from build123d import *

# Parameters (mm, degrees)
BOSS_EXTRUDE1_DEPTH = 5
FILLET1_R           = 40
FILLET2_R           = 1
SKETCH2_R           = 3
CUT_EXTRUDE1_DEPTH  = 1192.271634267


with BuildPart() as part:
    # Sketch1 → Boss-Extrude1 (new body)
    with BuildSketch(Plane.XY):
        Polygon((0, 0), (230, 0), (600.444279957, 1040), align=None)
    extrude(amount=BOSS_EXTRUDE1_DEPTH)

    # Fillet1
    fillet1_edges = [part.edges().sort_by_distance(p)[0] for p in [
        (230, 0, 2.5),
    ]]
    fillet(fillet1_edges, radius=FILLET1_R)

    # Fillet2
    fillet2_edges = [part.edges().sort_by_distance(p)[0] for p in [
        (600.444279957, 1040, 2.5),
    ]]
    fillet(fillet2_edges, radius=FILLET2_R)

    # Sketch2 → Cut-Extrude1 (cut, through all)
    with BuildSketch(Plane.XY.offset(5)):
        with Locations((249.147691634, 97.758565682)):
            Circle(SKETCH2_R)
        with Locations((273.494533389, 161.250543889)):
            Circle(SKETCH2_R)
        with Locations((515.885480129, 842.044902128)):
            Circle(SKETCH2_R)
        with Locations((540.232321884, 905.536880334)):
            Circle(SKETCH2_R)
    extrude(amount=-CUT_EXTRUDE1_DEPTH, mode=Mode.SUBTRACT)


solid = part.part
Can you work these out from the model? Positions are in its coordinate system, mm. Give positions to 0.01 mm unless a question says otherwise; leave off trailing zeros. Loops run counter-clockwise (first coordinate to the right, second up) from the corner with the lowest first, then second, coordinate; pieces in that order, holes last. Notation, with made-up numbers: (-16, 1) -> (-8, 1) arc R13 ccw to (-8, 21) -> close; hole circle Ø11 at (-8, -19.5). An arc over 180 degrees is marked (long way). Return JSON: item names as keys, results as strings.
Q1. I want a section at C-C, the plane x = 415.5. List the corners of the cut face in (y, z) for me, then the cut area to 3 significant figures.
Checks:
{"outline": "(520.78, 0) -> (719.67, 0) -> (719.67, 5) -> (520.78, 5) -> close", "area": "994 mm2"}
Q2. For pin 1 Ø3.5 at (x, y) = (515.89, 842.04) entering from +Z, with a flat end and sliding along its axis, tell me the tip position at first contact or that it passes through.
Checks:
{"pin 1": "passes through"}
Q3. I want a section at B-B, the plane y = 382. List the corners of the cut face in (x, z) for me.
Checks:
{"outline": "(220.55, 0) -> (366.07, 0) -> (366.07, 5) -> (220.55, 5) -> close"}
Q4. I need wall thicknesses on probe 1 along X at (y, z) = (380, 2.3); probe 2 along X at (y, z) = (729, 0.6); probe 3 along Y at (x, z) = (46, 0.3). Which ranges of each line are inside material? Lowest first, please.
Checks:
{"probe 1": "x = 219.39 to 365.35", "probe 2": "x = 420.89 to 489.67", "probe 3": "y = 0 to 79.67"}
Q5. I want a section at A-A, the plane z = 3.75. List the corners of the cut face in (x, y) for me.
Checks:
{"outline": "(0, 0) -> (201.79, 0) arc R40 ccw to (239.47, 26.58) -> (596.76, 1029.64) arc R1 ccw to (594.95, 1030.48) -> close; hole circle Ø6 at (249.15, 97.76); hole circle Ø6 at (273.49, 161.25); hole circle Ø6 at (515.89, 842.04); hole circle Ø6 at (540.23, 905.54)"}
